from build123d import *

# Parameters (mm, degrees)
SKETCH1_W               = 67
SKETCH1_H               = 35
BOSS_EXTRUDE1_DEPTH     = 4
CUT_EXTRUDE1_DEPTH      = 1
SKETCH3_W               = 67
SKETCH3_H               = 15
BOSS_EXTRUDE2_DEPTH     = 4
SKETCH4_W               = 38
SKETCH4_H               = 12
CUT_EXTRUDE2_DEPTH      = 10
SKETCH7_W               = 3.441650955
SKETCH7_H               = 28.44
CUT_EXTRUDE3_DEPTH      = 10
CHAMFER1_SIZE           = 1.5
CUT_EXTRUDE4_DEPTH      = 1.5
SKETCH5_W               = 35
SKETCH5_H               = 12
BOSS_EXTRUDE4_DEPTH     = 1.5
SKETCH9_R               = 1.925
SKETCH9_W               = 20.25
SKETCH9_H               = 20.25
CUT_EXTRUDE5_DEPTH      = 1.25
CUT_EXTRUDE6_DEPTH      = 6.6
CUT_EXTRUDE6_DEPTH_BACK = 6.6
SKETCH10_R              = 2.625
FILLET4_R               = 2
SKETCH11_W              = 12.25
SKETCH11_H              = 12.25
CUT_EXTRUDE8_DEPTH      = 0.5
SKETCH13_W              = 14.674904748
SKETCH13_H              = 14.674904748
SKETCH13_W_2            = 12.25
SKETCH13_H_2            = 12.25
BOSS_EXTRUDE5_DEPTH     = 1.5
FILLET5_R               = 1.25
FILLET6_R               = 1.25
SKETCH14_W              = 20.25
SKETCH14_H              = 1.651849009
CUT_EXTRUDE9_DEPTH      = 1.5


with BuildPart() as part:
    # Sketch1 → Boss-Extrude1 (new body)
    with BuildSketch(Plane(origin=(0, 0, 0), x_dir=(1, 0, 0), z_dir=(0, 1, 0))):
        Rectangle(SKETCH1_W, SKETCH1_H)
    extrude(amount=BOSS_EXTRUDE1_DEPTH)

    # Sketch2 → Cut-Extrude1 (cut)
    with BuildSketch(Plane(origin=(0, 4, 0), x_dir=(1, 0, 0), z_dir=(0, 1, 0))):
        Polygon((-27.51, 14.22), (27.419266745, 14.22), (33.5, 14.22), (33.5, -14.22), (30.165301507, -14.22), (-27.51, -14.22), align=None)
    extrude(amount=-CUT_EXTRUDE1_DEPTH, mode=Mode.SUBTRACT)

    # Sketch3 → Boss-Extrude2 (add)
    with BuildSketch(Plane(origin=(0, 4, 0), x_dir=(1, 0, 0), z_dir=(0, 1, 0))):
        with Locations((0, -25)):
            Rectangle(SKETCH3_W, SKETCH3_H)
    extrude(amount=-BOSS_EXTRUDE2_DEPTH)

    # Sketch4 → Cut-Extrude2 (cut)
    with BuildSketch(Plane(origin=(0, 4, 0), x_dir=(1, 0, 0), z_dir=(0, 1, 0))):
        with Locations((14.5, -23.36)):
            Rectangle(SKETCH4_W, SKETCH4_H)
    extrude(amount=-CUT_EXTRUDE2_DEPTH, mode=Mode.SUBTRACT)

    # Sketch7 → Cut-Extrude3 (cut)
    with BuildSketch(Plane(origin=(0, 3, 0), x_dir=(1, 0, 0), z_dir=(0, 1, 0))):
        with Locations((31.779174522, 0)):
            Rectangle(SKETCH7_W, SKETCH7_H)
    extrude(amount=-CUT_EXTRUDE3_DEPTH, mode=Mode.SUBTRACT)

    # Chamfer1
    chamfer1_edges = [part.edges().sort_by_distance(p)[0] for p in [
        (30.058349045, 1.5, 14.22),
        (30.058349045, 1.5, -14.22),
    ]]
    chamfer(chamfer1_edges, length=CHAMFER1_SIZE)

    # Sketch8 → Cut-Extrude4 (cut)
    with BuildSketch(Plane.XZ):
        with BuildLine():
            Line((30.058349045, 8.95), (1.508349045, 8.95))
            Line((1.508349045, 8.95), (1.508349045, 6.432050808))
            ThreePointArc((1.508349045, 6.432050808), (2.903992969, 6.022875656), (3.508349045, 4.7))
            Line((3.508349045, 4.7), (3.508349045, -4.7))
            ThreePointArc((3.508349045, -4.7), (2.903992969, -6.022875656), (1.508349045, -6.432050808))
            Line((1.508349045, -6.432050808), (1.508349045, -8.95))
            Line((1.508349045, -8.95), (30.058349045, -8.95))
            Line((30.058349045, -8.95), (30.058349045, 8.95))
        make_face()
    extrude(amount=-CUT_EXTRUDE4_DEPTH, mode=Mode.SUBTRACT)

    # Sketch5 → Boss-Extrude4 (add)
    with BuildSketch(Plane.XZ):
        with Locations((13, 23.36)):
            Rectangle(SKETCH5_W, SKETCH5_H)
    extrude(amount=-BOSS_EXTRUDE4_DEPTH)

    # Sketch9 → Cut-Extrude5 (cut)
    with BuildSketch(Plane.XZ):
        with Locations((-6.354971576, 21.536411907)):
            Circle(SKETCH9_R)
        with Locations((-26.604971576, 21.536411907)):
            Circle(SKETCH9_R)
        with Locations((-16.479971576, 21.536411907)):
            Rectangle(SKETCH9_W, SKETCH9_H)
        with BuildLine():
            ThreePointArc((-24.679971576, 21.536411907), (-25.243791022, 22.897592461), (-26.604971576, 23.461411907))
            Line((-26.604971576, 23.461411907), (-26.604971576, 19.611411907))
            ThreePointArc((-26.604971576, 19.611411907), (-25.243791022, 20.175231353), (-24.679971576, 21.536411907))
        make_face()
        with BuildLine():
            Line((-26.604971576, 19.611411907), (-26.604971576, 23.461411907))
            ThreePointArc((-26.604971576, 23.461411907), (-28.529971576, 21.536411907), (-26.604971576, 19.611411907))
        make_face()
        with BuildLine():
            ThreePointArc((-4.429971576, 21.536411907), (-4.993791022, 22.897592461), (-6.354971576, 23.461411907))
            Line((-6.354971576, 23.461411907), (-6.354971576, 19.611411907))
            ThreePointArc((-6.354971576, 19.611411907), (-4.993791022, 20.175231353), (-4.429971576, 21.536411907))
        make_face()
        with BuildLine():
            Line((-6.354971576, 19.611411907), (-6.354971576, 23.461411907))
            ThreePointArc((-6.354971576, 23.461411907), (-8.279971576, 21.536411907), (-6.354971576, 19.611411907))
        make_face()
    extrude(amount=-CUT_EXTRUDE5_DEPTH, mode=Mode.SUBTRACT)

    # Sketch10 → Cut-Extrude6 (cut, two sides: drawn at the far end of the back side and taken through both)
    with BuildSketch(Plane.XZ.offset(-1.25).offset(-CUT_EXTRUDE6_DEPTH_BACK)):
        with Locations((-16.479971576, 31.661411907)):
            Circle(SKETCH10_R)
    extrude(amount=CUT_EXTRUDE6_DEPTH + CUT_EXTRUDE6_DEPTH_BACK, mode=Mode.SUBTRACT)

    # Fillet4
    fillet4_edges = [part.edges().sort_by_distance(p)[0] for p in [
        (-18.967419065, 2, 32.5),
        (-13.992524087, 2, 32.5),
    ]]
    fillet(fillet4_edges, radius=FILLET4_R)

    # Sketch11 → Cut-Extrude8 (cut)
    with BuildSketch(Plane(origin=(0, 4, 0), x_dir=(1, 0, 0), z_dir=(0, 1, 0))):
        with Locations((-26.162547626, -23.36)):
            Rectangle(SKETCH11_W, SKETCH11_H)
    extrude(amount=-CUT_EXTRUDE8_DEPTH, mode=Mode.SUBTRACT)

    # Sketch13 → Boss-Extrude5 (add)
    with BuildSketch(Plane(origin=(0, 4, 0), x_dir=(1, 0, 0), z_dir=(0, 1, 0))):
        with Locations((-26.162547626, -23.36)):
            Rectangle(SKETCH13_W, SKETCH13_H)
        with Locations((-26.162547626, -23.36)):
            Rectangle(SKETCH13_W_2, SKETCH13_H_2, mode=Mode.SUBTRACT)
    extrude(amount=BOSS_EXTRUDE5_DEPTH)

    # Fillet5
    # the kernel refuses this fillet: 1.25 mm, written as the material it takes off along each edge
    with BuildSketch(Plane(origin=(-18.825095252, 4, 16.022547626), x_dir=(0, 0, 1), z_dir=(0, 1, 0)), Plane(origin=(-18.825095252, 4, 30.697452374), x_dir=(-1, 0, 0), z_dir=(0, 1, 0))) as fillet5_piece_1:
        with BuildLine():
            CenterArc((FILLET5_R, -FILLET5_R), FILLET5_R, 90, 90)
            Line((0, -FILLET5_R), (0, 0))
            Line((0, 0), (FILLET5_R, 0))
        make_face()
    extrude(amount=4.625, mode=Mode.SUBTRACT)

    # Fillet6
    fillet6_edges = [part.edges().sort_by_distance(p)[0] for p in [
        (-33.5, 2, 32.5),
        (33.5, 2, 32.5),
        (-33.5, 2, -17.5),
        (33.5, 2, -17.5),
    ]]
    fillet(fillet6_edges, radius=FILLET6_R)

    # Sketch14 → Cut-Extrude9 (cut)
    with BuildSketch(Plane.XZ.offset(-1.25)):
        with Locations((-16.479971576, 32.487336412)):
            Rectangle(SKETCH14_W, SKETCH14_H)
    extrude(amount=CUT_EXTRUDE9_DEPTH, mode=Mode.SUBTRACT)


solid = part.part
Work out the finished part from the listing and answer in its coordinate system (mm). A direction names the side the tool comes from. Give positions to 0.01 mm unless a question says otherwise; leave off trailing zeros. Order: outer loops, then holes, each group sorted by start corner. A loop starts at its lowest first (then second) coordinate and runs counter-clockwise, first axis right, second up. Notation, with made-up numbers: (14, -37.5) -> (27, -37.5) arc R33 cw to (27, -0.5) -> close; hole circle Ø10 at (-7, 61). An arc over 180 degrees is marked (long way). One line per item, written item: value.
Item 1: Flat-ended cylindrical pins translate along their axes: P1, Ø1.6, axis at y = 0.5, z = 8, coming from the +X side; P2, Ø3.5, axis at x = 11.5, z = 26, coming from the +Y side; P3, Ø5, axis at x = -26.5, z = 11, coming from the +Y side. Find the tip coordinate at first contact, or state that the pin passes through.
Answer sheet:
P1: x = 1.51
P2: y = 1.5
P3: y = 4
Item 2: Find section B-B, the plane z = 25. Give the vertices of the cut face in (x, y), plus the area to 3 significant figures.
Answer sheet:
outline: (-33.5, 0) -> (-26.6, 0) -> (-26.6, 1.25) -> (-6.35, 1.25) -> (-6.35, 0) -> (30.5, 0) -> (30.5, 1.5) -> (-4.5, 1.5) -> (-4.5, 4) -> (-18.83, 4) -> (-18.83, 5.5) -> (-20.04, 5.5) -> (-20.04, 3.5) -> (-32.29, 3.5) -> (-32.29, 5.5) -> (-33.5, 5.5) -> close
area: 141 mm²
Item 3: Determine the mould class of faces 6 (the flat face through (-27, 5, 16.023)), 7 (the flat face through (0, 0, 8)), 8 (the flat face through (-20.038, 4, 23)) for opening direction Z: released by +Z, released by -Z, zero draft, split by the parting line, or undercut.
Answer sheet:
face 6: released by -Z
face 7: zero draft
face 8: undercut
Item 4: Find section C-C, the plane y = 2.3. Give the vertices of the cut face in (x, z) (3 decimals).
Answer sheet:
outline: (-33.5, -16.25) arc R1.25 ccw to (-32.25, -17.5) -> (32.25, -17.5) arc R1.25 ccw to (33.5, -16.25) -> (33.5, -14.22) -> (31.558, -14.22) -> (30.058, -12.72) -> (30.058, 12.72) -> (31.558, 14.22) -> (33.5, 14.22) -> (33.5, 17.36) -> (-4.5, 17.36) -> (-4.5, 29.36) -> (33.5, 29.36) -> (33.5, 31.25) arc R1.25 ccw to (32.25, 32.5) -> (-12.003, 32.5) arc R2 ccw to (-13.939, 31.002) arc R2.625 cw to (-19.021, 31.002) arc R2 ccw to (-20.957, 32.5) -> (-32.25, 32.5) arc R1.25 ccw to (-33.5, 31.25) -> close
Item 5: Find section D-D, the plane z = -8. Give the vertices of the cut face in (x, y), plus the area to 3 significant figures.
Answer sheet:
outline: (-33.5, 0) -> (1.51, 0) -> (1.51, 1.5) -> (30.06, 1.5) -> (30.06, 3) -> (-27.51, 3) -> (-27.51, 4) -> (-33.5, 4) -> close
area: 154 mm²
Item 6: A tool of negligible diameter and unlimited length cuts with its end or side. For faces 1 (the flat face through (16, 1.5, 0)), 2 (the flat face through (2, 3, 0)), 3 (the cylindrical face through (-28.53, 0.62, 21.58)), 4 (the flat face through (-18.825, 5, 23)), 5 (the flat face through (30.5, 1, 23)), from which of +Z, -Z, +X, -X, +Y, -Y can it reach the whole face along a straight path? Write none if from no direction.
Answer sheet:
face 1: +X, -Y
face 2: +X, +Y
face 3: -Y
face 4: +Z, -Z, +X, +Y
face 5: +X, +Y, -Y
Item 7: Find section A-A, the plane x = -11. Give the vertices of the cut face in (y, z), plus the area to 3 significant figures.
Answer sheet:
outline: (0, -17.5) -> (4, -17.5) -> (4, -14.22) -> (3, -14.22) -> (3, 14.22) -> (4, 14.22) -> (4, 32.5) -> (1.25, 32.5) -> (1.25, 11.41) -> (0, 11.41) -> close
area: 145 mm²
Item 8: Straight lines are drawn through the part: probe 1 along Z at (x, y) = (28, 2.2); probe 2 along Z at (x, y) = (20.5, 3.6); probe 3 along Z at (x, y) = (-9, 3.15). For each, find the intervals that lie inside material, in ascending order.
Answer sheet:
probe 1: -17.5 to 17.36, 29.36 to 32.5
probe 2: -17.5 to -14.22, 14.22 to 17.36, 29.36 to 32.5
probe 3: -17.5 to -14.22, 14.22 to 32.5
